from build123d import *

# Parameters (mm, degrees)
SKETCH1_R           = 12.7
BOSS_EXTRUDE1_DEPTH = 25.4
SKETCH2_R           = 2.5527
CUT_EXTRUDE1_DEPTH  = 26.4
SKETCH3_R           = 6.35
CUT_EXTRUDE2_DEPTH  = 19.05
CHAMFER1_SIZE       = 2.54
SKETCH4_R           = 2.5527
CUT_EXTRUDE3_DEPTH  = 19.05


with BuildPart() as part:
    # Sketch1 → Boss-Extrude1 (new body)
    with BuildSketch(Plane.XY):
        Circle(SKETCH1_R)
    extrude(amount=BOSS_EXTRUDE1_DEPTH)

    # Sketch2 → Cut-Extrude1 (cut, through all)
    with BuildSketch(Plane.XY.offset(25.4)):
        Circle(SKETCH2_R)
    extrude(amount=-CUT_EXTRUDE1_DEPTH, mode=Mode.SUBTRACT)

    # Sketch3 → Cut-Extrude2 (cut)
    with BuildSketch(Plane.XY.offset(25.4)):
        Circle(SKETCH3_R)
    extrude(amount=-CUT_EXTRUDE2_DEPTH, mode=Mode.SUBTRACT)

    # Chamfer1
    chamfer1_edges = [part.edges().sort_by_distance(p)[0] for p in [
        (-12.7, 0, 25.4),
    ]]
    chamfer(chamfer1_edges, length=CHAMFER1_SIZE)

    # Sketch4 → Cut-Extrude3 (cut)
    with BuildSketch(Plane(origin=(0, 0, 0), x_dir=(1, 0, 0), z_dir=(0, 1, 0))):
        with Locations((0, -19.05)):
            Circle(SKETCH4_R)
    extrude(amount=-CUT_EXTRUDE3_DEPTH, mode=Mode.SUBTRACT)


solid = part.part
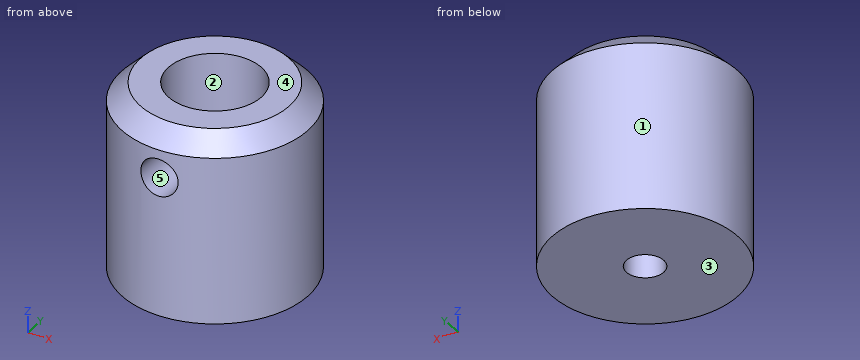
Could you check a few things on this model? Use its own coordinates, in mm. Face numbers are marked on the shaded views. A direction names the side the tool comes from. Round coordinates to 2 decimals unless told otherwise and drop trailing zeros. Order: outer loops, then holes, each group sorted by start corner. A loop starts at its lowest first (then second) coordinate and runs counter-clockwise, first axis right, second up.
(1) If we mould it in two halves opening along Y, with no side actions, what happens to the marked faces 1, 2 and 3? For each: released by +Y, released by -Y, zero draft, split by the parting line, or undercut.
Response values:
face 1: split by the parting line
face 2: undercut
face 3: zero draft
(2) Please list where these lines run through material, in increasing order: line 1 along Z through (x, y) = (0, -9.75); line 2 along Y through (x, z) = (0, 4.25); line 3 along Y through (x, z) = (0, 11.75).
Response values:
line 1: z = 0 to 16.5, 21.6 to 25.4
line 2: y = -12.7 to -2.55, 2.55 to 12.7
line 3: y = -12.7 to -6.35, 6.35 to 12.7
(3) Imagine slicing it at A-A (x = 0). Write out the boundary of the cut face in (y, z).
Response values:
outline: (-12.7, 0) - (-2.55, 0) - (-2.55, 6.35) - (-6.35, 6.35) - (-6.35, 16.5) - (-12.7, 16.5) - close; (-12.7, 21.6) - (-6.35, 21.6) - (-6.35, 25.4) - (-10.16, 25.4) - (-12.7, 22.86) - close; (2.55, 0) - (12.7, 0) - (12.7, 22.86) - (10.16, 25.4) - (6.35, 25.4) - (6.35, 6.35) - (2.55, 6.35) - close
(4) Which directions (+Z, -Z, +X, -X, +Y, -Y) give clear straight access to the entire face, cutting with the end or side of a thin tool? Please do the marked faces 4 and 5.
Response values:
face 4: +Z, +X, -X, +Y, -Y
face 5: -Y
(5) Imagine slicing it at C-C (z = 11). Write out the boundary of the cut face in (x, y), plus the area to 3 significant figures.
Response values:
outline: circle Ø25.4 at (0, 0); hole circle Ø12.7 at (0, 0)
area: 380 mm2
(6) Imagine slicing it at D-D (z = 4). Write out the boundary of the cut face in (x, y).
Response values:
outline: circle Ø25.4 at (0, 0); hole circle Ø5.11 at (0, 0)
(7) Imagine slicing it at B-B (y = 0). Write out the boundary of the cut face in (x, z).
Response values:
outline: (-12.7, 0) - (-2.55, 0) - (-2.55, 6.35) - (-6.35, 6.35) - (-6.35, 25.4) - (-10.16, 25.4) - (-12.7, 22.86) - close; (2.55, 0) - (12.7, 0) - (12.7, 22.86) - (10.16, 25.4) - (6.35, 25.4) - (6.35, 6.35) - (2.55, 6.35) - close
(8) I'm going to push flat-ended pins straight in: pin 1 (4 mm diameter, centred on x = 0, z = 19.05, fed in from -Y); pin 2 (12 mm diameter, centred on y = 9.5, z = 4, fed in from -X); pin 3 (5 mm diameter, centred on y = -7.5, z = 4.5, fed in from -X). Where does each tip first touch, or does it pass through?
Response values:
pin 1: stops at y = 6.03
pin 2: stops at x = -12.21
pin 3: stops at x = -11.67
